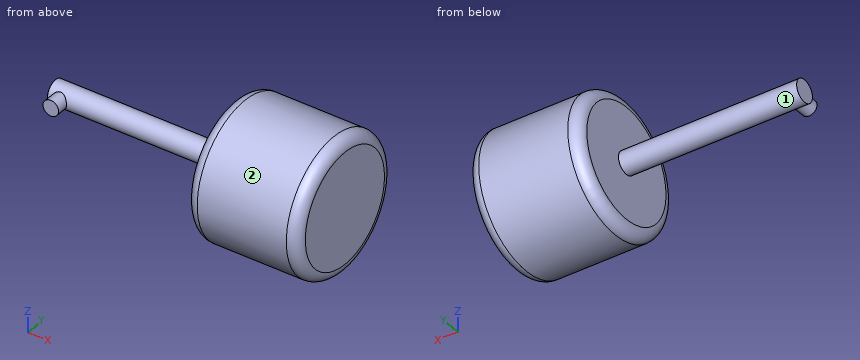
from build123d import *

# Parameters (mm, degrees)
F0_R     = 30
F1_DEPTH = 50
F2_R     = 5
F3_DEPTH = 80
F4_R     = 3.5
F5_DEPTH = 10
F6_R     = 5


with BuildPart() as f1:
    # F0 (on Right) → F1 (new body)
    with BuildSketch(Plane.YZ):
        Circle(F0_R)
    extrude(amount=F1_DEPTH)

    # F2 (on Right) → F3 (join)
    with BuildSketch(Plane.YZ):
        Circle(F2_R)
    extrude(amount=-F3_DEPTH)

    # F4 (on Front) → F5 (join)
    with BuildSketch(Plane.XZ):
        with Locations((-75, 0)):
            Circle(F4_R)
    extrude(amount=F5_DEPTH)

    # F6
    f6_edges = [f1.edges().sort_by_distance(p)[0] for p in [
        (50, -30, 0),
        (0, -30, 0),
    ]]
    fillet(f6_edges, radius=F6_R)


solid = f1.part
CAD build for the part. Positions are in the model's coordinates, mm. Face numbers are marked on the shaded views. A direction names the side the tool comes from. Round coordinates to 2 decimals unless told otherwise and drop trailing zeros. Write each loop counter-clockwise with the first axis right and the second up, starting at its lowest first coordinate (ties: lowest second). Pieces come first, ordered by that corner, then holes. Notation, with made-up numbers: M -11.5,81 L 27.5,81 A18 cw 27.5,113 Z; hole C -8,-34 d1. An arc over 180 degrees is marked long. Put each result on its own line as item: value. Start each with the question number.
1) Drill centre lines: probe 1 along X at (y, z) = (-17, -18); probe 2 along Z at (x, y) = (-7, 0.5); probe 3 along Y at (x, z) = (30, 26). Where is each one in solid material? Low to high. Write a range as [from, to].
2) Saw through at D-D, the plane x = -14. Write the cut outline in (y, z), and give its area (3 significant figures).
3) Pin check, flat tips, straight feed: pin 1 Ø10 at (y, z) = (-21, -3.5) entering from -X; pin 2 Ø2 at (x, z) = (-76.5, 1) entering from -Y; pin 3 Ø10 at (x, z) = (-50.5, -1.5) entering from +Y; pin 4 Ø15 at (y, z) = (-9.5, -4.5) entering from -X. Stop position of each tip, or through.
4) 3-axis set-ups, long thin cutter, end or side, ignore diameter. For the marked faces 1 and 2: which of +Z, -Z, +X, -X, +Y, -Y reach the whole face in a straight line?
5) Saw through at C-C, the plane x = -75. Write the cut outline in (y, z).
6) Saw through at B-B, the plane y = 0. Write the cut outline in (x, z), and give its area (3 significant figures).
7) Saw through at A-A, the plane z = 0. Write the cut outline in (x, y).
Resolved:
1. probe 1: [0, 50]
1. probe 2: [-4.97, 4.97]
1. probe 3: [-14.97, 14.97]
2. outline: C 0,0 d10
2. area: 78.5 mm²
3. pin 1: x = 0
3. pin 2: y = -10
3. pin 3: y = 5
3. pin 4: x = -80
4. face 1: none
4. face 2: +X, -X
5. outline: M -10,-3.5 L -3.57,-3.5 A5 ccw long -3.57,3.5 L -10,3.5 Z
6. outline: M -80,-5 L 0,-5 L 0,-25 A5 ccw 5,-30 L 45,-30 A5 ccw 50,-25 L 50,25 A5 ccw 45,30 L 5,30 A5 ccw 0,25 L 0,5 L -80,5 Z
6. area: 3,780 mm²
7. outline: M -80,-5 L -78.5,-5 L -78.5,-10 L -71.5,-10 L -71.5,-5 L 0,-5 L 0,-25 A5 ccw 5,-30 L 45,-30 A5 ccw 50,-25 L 50,25 A5 ccw 45,30 L 5,30 A5 ccw 0,25 L 0,5 L -80,5 Z
